```python
from build123d import *

# Parameters (mm, degrees)
BOSS_EXTRUDE1_DEPTH = 3.175
FILLET1_R           = 1


with BuildPart() as part:
    # Sketch1 → Boss-Extrude1 (new body)
    with BuildSketch(Plane.XY):
        Polygon((-40.925, -23.815), (-15, -23.815), (-15, -26.99), (15, -26.99), (15, -23.815), (40.925, -23.815), (40.925, 23.815), (15, 23.815), (15, 26.99), (-15, 26.99), (-15, 23.815), (-40.925, 23.815), align=None)
    extrude(amount=BOSS_EXTRUDE1_DEPTH)

    # Fillet1
    fillet1_edges = [part.edges().sort_by_distance(p)[0] for p in [
        (-15, -26.99, 1.5875),
        (15, -26.99, 1.5875),
        (15, 26.99, 1.5875),
        (-15, 26.99, 1.5875),
    ]]
    fillet(fillet1_edges, radius=FILLET1_R)


solid = part.part
```
CAD build for the part. Positions are in the model's coordinates, mm. A direction names the side the tool comes from. Round coordinates to 2 decimals unless told otherwise and drop trailing zeros. Loops run counter-clockwise (first coordinate to the right, second up) from the corner with the lowest first, then second, coordinate; pieces in that order, holes last. Notation, with made-up numbers: M 46,63.25 L 72,63.25 A8 ccw 72,69.25 Z; hole C 34.25,56.25 d11. An arc over 180 degrees is marked long. Use a Markdown table: item, result. Add a question column.
(1) Cut at B-B (x = 21). Give the cut face in (y, z) (3 decimals).
(2) Flat gauge pins, fed straight in: pin 1 (1.1 mm diameter, centred on y = 24.5, z = 1, fed in from +X); pin 2 (1.6 mm diameter, centred on x = -33.5, z = 2, fed in from -Y) (3 decimals); pin 3 (0.7 mm diameter, centred on y = 25, z = 1.5, fed in from -X); pin 4 (10 mm diameter, centred on x = -23.5, y = 17, fed in from -Z). Where does each tip first touch, or does it go through?
(3) Cut at A-A (z = 2.2). Give the cut face in (x, y) (3 decimals).
(4) Drill centre lines: line 1 (Y direction, x = 19.5, z = 2.45) (3 decimals); line 2 (X direction, y = 24, z = 1.1). Where is each one in solid material? Low to high.
(5) Which spindle directions (+Z, -Z, +X, -X, +Y, -Y) get a long thin tool onto all of the face, cutting with end or side? Do faces 4 (the face through (-28, -23.815, 2)), 5 (the face through (15, 25, 2)), 6 (the face through (15, -25, 2)), 7 (the face through (-28, 23.815, 2)). Say none if no direction does.
(6) Pull direction Z, two halves, no side cores. Call faces 1 (the face through (-1, 0, 0)), 2 (the face through (-1, 0, 3.175)), 3 (the face through (0, -26.99, 2)): +Z half, -Z half, draft (parallel to the pull), parting line (faces both ways), or undercut.
Geometry says:
| question | item | result |
|---|---|---|
| 1 | outline | M -23.815,0 L 23.815,0 L 23.815,3.175 L -23.815,3.175 Z |
| 2 | pin 1 | stops at x = 15 |
| 2 | pin 2 | stops at y = -23.815 |
| 2 | pin 3 | stops at x = -15 |
| 2 | pin 4 | stops at z = 0 |
| 3 | outline | M -40.925,-23.815 L -15,-23.815 L -15,-25.99 A1 ccw -14,-26.99 L 14,-26.99 A1 ccw 15,-25.99 L 15,-23.815 L 40.925,-23.815 L 40.925,23.815 L 15,23.815 L 15,25.99 A1 ccw 14,26.99 L -14,26.99 A1 ccw -15,25.99 L -15,23.815 L -40.925,23.815 Z |
| 4 | line 1 | y = -23.815 to 23.815 |
| 4 | line 2 | x = -15 to 15 |
| 5 | face 4 | +Z, -Z, -X, -Y |
| 5 | face 5 | +Z, -Z, +X, +Y |
| 5 | face 6 | +Z, -Z, +X, -Y |
| 5 | face 7 | +Z, -Z, -X, +Y |
| 6 | face 1 | -Z half |
| 6 | face 2 | +Z half |
| 6 | face 3 | draft |
